The model under review builds one solid part; all positions refer to its coordinate system, in mm. Round coordinates to 2 decimals unless told otherwise and drop trailing zeros. Write each loop counter-clockwise with the first axis right and the second up, starting at its lowest first coordinate (ties: lowest second). Pieces come first, ordered by that corner, then holes. Notation, with made-up numbers: (55, -24.75) - (81, -24.75) arc R31 ccw to (81, 12.25) - close; hole circle Ø4 at (63.25, 61). An arc over 180 degrees is marked (long way). Return JSON: item names as keys, results as strings.
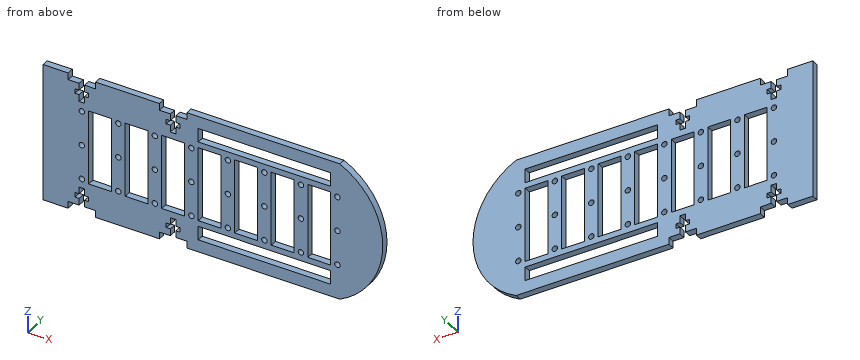
from build123d import *

# Parameters (mm, degrees)
BOSS_EXTRUDE1_DEPTH  = 3.81
CUT_EXTRUDE8_DEPTH   = 103.498384567
MIRROR6_COPY_1_DEPTH = 103.498384567
SKETCH5_R            = 1.524
CUT_EXTRUDE2_DEPTH   = 103.498384567
LPATTERN1_COUNT      = 3
LPATTERN1_PITCH      = 19.05
LPATTERN1_COUNT_DIR2 = 8
LPATTERN1_PITCH_DIR2 = 20.32
SKETCH6_W            = 12.7
SKETCH6_H            = 41.148
CUT_EXTRUDE5_DEPTH   = 103.498384567
LPATTERN2_COUNT      = 3
LPATTERN2_PITCH      = 20.32
LPATTERN3_COUNT      = 5
LPATTERN3_PITCH      = 20.32
SKETCH7_W            = 73.66
SKETCH7_H            = 7.62
CUT_EXTRUDE6_DEPTH   = 103.498384567


with BuildPart() as part:
    # Sketch2 → Boss-Extrude1 (new body)
    with BuildSketch(Plane(origin=(0, 0, 0), x_dir=(1, 0, 0), z_dir=(0, 1, 0))):
        with BuildLine():
            Line((-93.98, 38.1), (-93.98, -38.1))
            Line((-93.98, -38.1), (71.12, -38.1))
            ThreePointArc((71.12, -38.1), (95.077824642, 0), (71.12, 38.1))
            Line((71.12, 38.1), (-93.98, 38.1))
        make_face()
    extrude(amount=BOSS_EXTRUDE1_DEPTH)

    # Sketch9 → Cut-Extrude8 (cut, symmetric)
    with BuildSketch(Plane.XZ):
        Polygon((-80.01, 430.001486449), (-80.01, 38.1), (-80.01, 34.29), (-73.914, 34.29), (-73.914, 30.48), (-76.2, 30.48), (-76.2, 27.94), (-73.914, 27.94), (-73.914, 24.13), (-70.866, 24.13), (-70.866, 27.94), (-68.58, 27.94), (-68.58, 30.48), (-70.866, 30.48), (-70.866, 34.29), (-64.77, 34.29), (-64.77, 38.1), (-64.77, 430.001486449), (-64.77, 1213.804459348), (-80.01, 1213.804459348), align=None)
    cut_extrude8 = extrude(amount=CUT_EXTRUDE8_DEPTH, both=True, mode=Mode.SUBTRACT)

    # Mirror5: Cut-Extrude8 across plane
    add(cut_extrude8.mirror(Plane(origin=(-46.99, 0, 0), x_dir=(0, 0, 1), z_dir=(1, 0, 0))), mode=Mode.SUBTRACT)

    # Mirror6: Cut-Extrude8 across plane
    add(cut_extrude8.mirror(Plane.XY), mode=Mode.SUBTRACT)

    # Mirror6 copy 1 sketch → Mirror6 copy 1 (cut, symmetric)
    with BuildSketch(Plane(origin=(-93.98, 0, 0), x_dir=(-1, 0, 0), z_dir=(0, -1, 0))):
        Polygon((-80.01, 430.001486449), (-80.01, 38.1), (-80.01, 34.29), (-73.914, 34.29), (-73.914, 30.48), (-76.2, 30.48), (-76.2, 27.94), (-73.914, 27.94), (-73.914, 24.13), (-70.866, 24.13), (-70.866, 27.94), (-68.58, 27.94), (-68.58, 30.48), (-70.866, 30.48), (-70.866, 34.29), (-64.77, 34.29), (-64.77, 38.1), (-64.77, 430.001486449), (-64.77, 1213.804459348), (-80.01, 1213.804459348), align=None)
    extrude(amount=MIRROR6_COPY_1_DEPTH, both=True, mode=Mode.SUBTRACT)

    # Sketch5 → Cut-Extrude2 (cut, through all)
    with BuildSketch(Plane.XZ):
        with Locations(Location((-72.39, 19.05, 0), (0, 0, 270))):
            Circle(SKETCH5_R)
    cut_extrude2 = extrude(amount=-CUT_EXTRUDE2_DEPTH, mode=Mode.SUBTRACT)

    # LPattern1: Cut-Extrude2 3 × 8
    with Locations(*[(j * LPATTERN1_PITCH_DIR2, 0, -i * LPATTERN1_PITCH) for i in range(LPATTERN1_COUNT) for j in range(LPATTERN1_COUNT_DIR2) if (i, j) != (0, 0)]):
        add(cut_extrude2, mode=Mode.SUBTRACT)

    # Sketch6 → Cut-Extrude5 (cut, through all)
    with BuildSketch(Plane.XZ):
        with Locations((-21.59, 0)):
            Rectangle(SKETCH6_W, SKETCH6_H)
    cut_extrude5 = extrude(amount=-CUT_EXTRUDE5_DEPTH, mode=Mode.SUBTRACT)

    # LPattern2: Cut-Extrude5 ×3
    with Locations(*[(-i * LPATTERN2_PITCH, 0, 0) for i in range(1, LPATTERN2_COUNT)]):
        add(cut_extrude5, mode=Mode.SUBTRACT)

    # LPattern3: Cut-Extrude5 ×5
    with Locations(*[(i * LPATTERN3_PITCH, 0, 0) for i in range(1, LPATTERN3_COUNT)]):
        add(cut_extrude5, mode=Mode.SUBTRACT)

    # Sketch7 → Cut-Extrude6 (cut, through all)
    with BuildSketch(Plane.XZ):
        with Locations((29.21, 27.559)):
            Rectangle(SKETCH7_W, SKETCH7_H)
    cut_extrude6 = extrude(amount=-CUT_EXTRUDE6_DEPTH, mode=Mode.SUBTRACT)

    # Mirror3: Cut-Extrude6 across plane
    add(cut_extrude6.mirror(Plane.XY), mode=Mode.SUBTRACT)


solid = part.part
(1) Clearance check with flat-ended pins moving along their axes: pin 1 Ø1.5 at (y, z) = (1.5, -21) entering from +X; pin 2 Ø1.1 at (x, y) = (-19, 2) entering from +Z; pin 3 Ø1.9 at (y, z) = (2, 33) entering from +X. State where each tip first meets the part, or that it passes through.
Filled in:
{"pin 1": "stops at x = 89.91", "pin 2": "stops at z = 34.29", "pin 3": "stops at x = 80.37"}
(2) Add section A-A (x = -62). Write out the cut boundary in (y, z), plus the area to 3 significant figures.
Filled in:
{"outline": "(0, -38.1) - (3.81, -38.1) - (3.81, -20.57) - (0, -20.57) - close; (0, 20.57) - (3.81, 20.57) - (3.81, 38.1) - (0, 38.1) - close", "area": "134 mm2"}
(3) Wall thickness on line 1 (Z direction, x = 27.5, y = 2.3); line 2 (Z direction, x = 37, y = 1.35); line 3 (Z direction, x = -15.5, y = 1.75): over which ranges is each line inside the solid? List them lowest first.
Filled in:
{"line 1": "z = -38.1 to -31.37, -23.75 to 23.75, 31.37 to 38.1", "line 2": "z = -38.1 to -31.37, -23.75 to -20.57, 20.57 to 23.75, 31.37 to 38.1", "line 3": "z = -34.29 to -20.57, 20.57 to 34.29"}
(4) Add section B-B (z = 12). Give the number of separate pieces and of enclosed holes in the cut face, plus the area to 3 significant figures.
Filled in:
{"separate pieces": "8", "enclosed holes": "0", "area": "375 mm2"}
